from build123d import *

# Parameters (mm, degrees)
SALIENTE_EXTRUIR1_DEPTH = 130
CROQUIS3_R              = 7.332348419
CROQUIS3_R_2            = 6
CORTAR_EXTRUIR1_DEPTH   = 65
CROQUIS4_R              = 6
CROQUIS4_R_2            = 5
CORTAR_EXTRUIR2_DEPTH   = 27
CROQUIS5_R              = 5
CROQUIS5_R_2            = 4
CORTAR_EXTRUIR3_DEPTH   = 20
CROQUIS6_R              = 4
CROQUIS6_R_2            = 3
CORTAR_EXTRUIR4_DEPTH   = 7


with BuildPart() as part:
    # Croquis2 → Saliente-Extruir1 (new body)
    with BuildSketch(Plane(origin=(0, 0, 0), x_dir=(1, 0, 0), z_dir=(0, 1, 0))):
        Polygon((7.332348419, 0), (3.666174209, 6.35), (-3.666174209, 6.35), (-7.332348419, 0), (-3.666174209, -6.35), (3.666174209, -6.35), align=None)
    extrude(amount=SALIENTE_EXTRUIR1_DEPTH)

    # Croquis3 → Cortar-Extruir1 (cut)
    with BuildSketch(Plane(origin=(0, 130, 0), x_dir=(1, 0, 0), z_dir=(0, 1, 0))):
        Circle(CROQUIS3_R)
        with Locations(Location((0, 0, 0), (0, 0, 270))):
            Circle(CROQUIS3_R_2, mode=Mode.SUBTRACT)
    extrude(amount=-CORTAR_EXTRUIR1_DEPTH, mode=Mode.SUBTRACT)

    # Croquis4 → Cortar-Extruir2 (cut)
    with BuildSketch(Plane(origin=(0, 130, 0), x_dir=(1, 0, 0), z_dir=(0, 1, 0))):
        with Locations(Location((0, 0, 0), (0, 0, 270))):
            Circle(CROQUIS4_R)
        with Locations(Location((0, 0, 0), (0, 0, 270))):
            Circle(CROQUIS4_R_2, mode=Mode.SUBTRACT)
    extrude(amount=-CORTAR_EXTRUIR2_DEPTH, mode=Mode.SUBTRACT)

    # Croquis5 → Cortar-Extruir3 (cut)
    with BuildSketch(Plane(origin=(0, 130, 0), x_dir=(1, 0, 0), z_dir=(0, 1, 0))):
        with Locations(Location((0, 0, 0), (0, 0, 270))):
            Circle(CROQUIS5_R)
        with Locations(Location((0, 0, 0), (0, 0, 270))):
            Circle(CROQUIS5_R_2, mode=Mode.SUBTRACT)
    extrude(amount=-CORTAR_EXTRUIR3_DEPTH, mode=Mode.SUBTRACT)

    # Croquis6 → Cortar-Extruir4 (cut)
    with BuildSketch(Plane(origin=(0, 130, 0), x_dir=(1, 0, 0), z_dir=(0, 1, 0))):
        with Locations(Location((0, 0, 0), (0, 0, 270))):
            Circle(CROQUIS6_R)
        with Locations(Location((0, 0, 0), (0, 0, 270))):
            Circle(CROQUIS6_R_2, mode=Mode.SUBTRACT)
    extrude(amount=-CORTAR_EXTRUIR4_DEPTH, mode=Mode.SUBTRACT)


solid = part.part
Design review of the part built by this model. Coordinates are the model's own, in mm. A direction names the side the tool comes from. Round coordinates to 2 decimals unless told otherwise and drop trailing zeros. Write each loop counter-clockwise with the first axis right and the second up, starting at its lowest first coordinate (ties: lowest second). Pieces come first, ordered by that corner, then holes. Notation, with made-up numbers: (-33.5, -19.75) - (-12.5, -19.75) arc R16 ccw to (-12.5, -5.75) - close; hole circle Ø2 at (-24, -23). An arc over 180 degrees is marked (long way). Use a Markdown table: item, result. Add a question column.
1. Wall thickness on probe 1 along X at (y, z) = (96, 4.75); probe 2 along Y at (x, z) = (-2.25, -3.25); probe 3 along Y at (x, z) = (-6.5, 0.5): over which ranges is each line inside the solid? List them lowest first.
2. Mouldability with a two-part tool opening along X and no side actions: class faces 1 (the face through (5.525, 32.045, -3.131)), 2 (the face through (-3.905, 116.591, -0.867)), 3 (the face through (-5.474, 32.045, -3.219)), 4 (the face through (4, 103, -4)) as +X half, -X half, draft (parallel to the pull), parting line (faces both ways), or undercut.
3. We need section B-B (y = 36.5). State the section outline as (x, z) points.
4. We need section A-A (x = 0). State the section outline as (y, z) points, then the cut area to 3 significant figures.
5. Clearance check with flat-ended pins moving along their axes: pin 1 (2 mm diameter, centred on x = 4, z = 0.5, fed in from +Y); pin 2 (6 mm diameter, centred on y = 116.5, z = 5, fed in from -X); pin 3 (2 mm diameter, centred on x = -5, y = 29, fed in from -Z). State where each tip first meets the part, or that it passes through.
6. We need section C-C (y = 69). State the section outline as (x, z) points.
7. We need section D-D (y = 108.5). State the section outline as (x, z) points.
8. For faces 5 (the face through (-5.525, 32.045, 3.131)), 6 (the face through (-4.88, 106.55, -1.08)), list the 3-axis set-ups (+Z, -Z, +X, -X, +Y, -Y) from which the entire face can be reached by the end or side of a thin tool; tool diameter is ignored.
Output:
| question | item | result |
|---|---|---|
| 1 | probe 1 | x = -3.67 to 3.67 |
| 1 | probe 2 | y = 0 to 123 |
| 1 | probe 3 | y = 0 to 65 |
| 2 | face 1 | +X half |
| 2 | face 2 | parting line |
| 2 | face 3 | -X half |
| 2 | face 4 | draft |
| 3 | outline | (-7.33, 0) - (-3.67, -6.35) - (3.67, -6.35) - (7.33, 0) - (3.67, 6.35) - (-3.67, 6.35) - close |
| 4 | outline | (0, -6.35) - (65, -6.35) - (65, -6) - (103, -6) - (103, -5) - (110, -5) - (110, -4) - (123, -4) - (123, -3) - (130, -3) - (130, 3) - (123, 3) - (123, 4) - (110, 4) - (110, 5) - (103, 5) - (103, 6) - (65, 6) - (65, 6.35) - (0, 6.35) - close |
| 4 | area | 1,500 mm2 |
| 5 | pin 1 | stops at y = 123 |
| 5 | pin 2 | stops at x = -3.46 |
| 5 | pin 3 | stops at z = -5.77 |
| 6 | outline | circle Ø12 at (0, 0) |
| 7 | outline | circle Ø10 at (0, 0) |
| 8 | face 5 | +Z, -X, +Y, -Y |
| 8 | face 6 | +Y |
